Here's how the part is built. I have some questions about the finished solid (model axes, mm). A direction names the side the tool comes from. Give positions to 0.01 mm unless a question says otherwise; leave off trailing zeros. Loops run counter-clockwise (first coordinate to the right, second up) from the corner with the lowest first, then second, coordinate; pieces in that order, holes last.
Q1. If we section it at A-A (z = 0): Please give me the cut outline in (x, y), plus the area to 3 significant figures.
Q2. I need wall thicknesses on line 1 (Z direction, x = 6, y = -13); line 2 (X direction, y = -6.75, z = 9.5); line 3 (Y direction, x = 23.5, z = 13). Which ranges of each line are inside material? Lowest first, please.
Q3. If we section it at B-B (y = -14.5): Please give me the cut outline in (x, z).
Q4. Will these pins go through, and if not, where does the flat tip stop? P1, Ø4, axis at x = 6, z = 34, coming from the -Y side; P2, Ø0.9, axis at x = 23.5, y = 1.5, coming from the +Z side.
Q5. For faces 1 (the face through (-26, -10.8, -43.57)), 2 (the face through (0, -12, -42.5)), 3 (the face through (25.273, 1, 0)), 4 (the face through (20.273, 1, 0)), which set-ups out of +Z, -Z, +X, -X, +Y, -Y let a thin tool reach every point of the face, with its end or its side?
Q6. If we section it at D-D (y = 1.25): Please give me the cut outline in (x, z), plus the area to 3 significant figures.
Q7. If we section it at C-C (x = 13): Please give me the cut outline in (y, z).
Q8. We'd pull the mould along X, two halves only. Please class faces 5 (the face through (18.677, 1.479, -17.722)), 6 (the face through (-27, -25, 0)), 7 (the face through (-27.5, -11, 1)): +X half, -X half, draft (parallel to the pull), parting line (faces both ways), or undercut.
Autodesk Inventor part; units mm, degrees
ref_plane "YZ Plane" through (0, 0, 0) normal (1, 0, 0) x (0, 1, 0)
ref_plane "XZ Plane" through (0, 0, 0) normal (0, 1, 0) x (-1, 0, 0)
ref_plane "XY Plane" through (0, 0, 0) normal (0, 0, 1) x (1, 0, 0)
sketch "Sketch1" plane through (0, 0, 0) normal (0, 1, 0) x (-1, 0, 0)
  line L0 (22.5, 45) -> (-22.5, 45)
  line L1 (-27.5, 40) -> (-27.5, -40)
  line L2 (-22.5, -45) -> (22.5, -45)
  line L3 (27.5, -40) -> (27.5, 40)
  line L4 (27.5, 45) -> (-27.5, -45) construction
  line L5 (-27.5, 45) -> (27.5, -45) construction
  line L6 (0, 0) -> (17.6777, 17.6777) construction
  line L7 (0, 0) -> (25, 0) construction
  circle A0 centre (17.6777, 17.6777) radius 1
  line L8 (17.6777, 17.6777) -> (21.2132, 14.1421) construction
  arc A1 (21.2132, 14.1421) -> (14.1421, 21.2132) centre (17.6777, 17.6777) ccw construction
  circle A2 centre (0, 0) radius 20 construction
  line L9 (14.1421, 21.2132) -> (10.1575, 17.2286) construction
  arc A3 (-6.25, 18.9984) -> (6.25, 18.9984) centre (0, 0) ccw construction
  line L10 (21.2132, 14.1421) -> (17.2286, 10.1575) construction
  line L11 (-14.1421, 21.2132) -> (-10.1575, 17.2286) construction
  arc A4 (-14.1421, 21.2132) -> (-21.2132, 14.1421) centre (-17.6777, 17.6777) ccw construction
  line L12 (-21.2132, 14.1421) -> (-17.2286, 10.1575) construction
  circle A5 centre (-17.6777, 17.6777) radius 1
  line L13 (-21.2132, -14.1421) -> (-17.2286, -10.1575) construction
  arc A6 (-21.2132, -14.1421) -> (-14.1421, -21.2132) centre (-17.6777, -17.6777) ccw construction
  line L14 (-14.1421, -21.2132) -> (-10.1575, -17.2286) construction
  circle A7 centre (-17.6777, -17.6777) radius 1
  line L15 (14.1421, -21.2132) -> (10.1575, -17.2286) construction
  arc A8 (14.1421, -21.2132) -> (21.2132, -14.1421) centre (17.6777, -17.6777) ccw construction
  line L16 (21.2132, -14.1421) -> (17.2286, -10.1575) construction
  circle A9 centre (17.6777, -17.6777) radius 1
  line L17 (-20.273, 10) -> (-25.273, 10)
  line L18 (-25.273, 10) -> (-25.273, -10)
  line L19 (-25.273, -10) -> (-20.273, -10)
  line L20 (-20.273, -10) -> (-20.273, 10)
  line L21 (-20.273, 10) -> (-25.273, -10) construction
  line L22 (-25.273, 10) -> (-20.273, -10) construction
  line L23 (39.9497, 0) -> (-39.9497, 0)
  arc A10 (22.5, -45) -> (27.5, -40) centre (22.5, -40) ccw
  arc A11 (27.5, 40) -> (22.5, 45) centre (22.5, 40) ccw
  arc A12 (-22.5, 45) -> (-27.5, 40) centre (-22.5, 40) ccw
  arc A13 (-27.5, -40) -> (-22.5, -45) centre (-22.5, -40) ccw
  point P0 (-22.773, 0)
  point P1 (-22.773, 0)
  dimension "d0" = 55
  dimension "d1" = 90
  dimension "d4" = 25
  dimension "d5" = 45
  dimension "d6" = 2
  dimension "d7" = 5
  dimension "d8" = 360
  dimension "d9" = 5
  dimension "d10" = 20
  dimension "d18" = 5
extrude "Extrusion1" add sketch "Sketch1" along normal blind 3 contours A11 L3 L23 L20 L17 L18 L1 A12 L0 | L3 A10 L2 A13 L1 L23 L18 L19 L20
sketch "Sketch2" plane through (0, 0, 0) normal (0, -1, 0) x (1, 0, 0)
  line L0 (22.5, 45) -> (-22.5, 45)
  line L1 (-27.5, 40) -> (-27.5, -40)
  line L2 (-22.5, -45) -> (22.5, -45)
  line L3 (27.5, -40) -> (27.5, 40)
  line L4 (27.5, 45) -> (-27.5, -45) construction
  line L5 (-27.5, 45) -> (27.5, -45) construction
  line L6 (17, 42.5) -> (-17, 42.5)
  line L7 (-25, 34.5) -> (-25, -34.5)
  line L8 (-17, -42.5) -> (17, -42.5)
  line L9 (25, -34.5) -> (25, 34.5)
  line L10 (25, 42.5) -> (-25, -42.5) construction
  line L11 (-25, 42.5) -> (25, -42.5) construction
  arc A0 (25, 34.5) -> (17, 42.5) centre (17, 34.5) ccw
  arc A1 (17, -42.5) -> (25, -34.5) centre (17, -34.5) ccw
  arc A2 (-25, -34.5) -> (-17, -42.5) centre (-17, -34.5) ccw
  arc A3 (-17, 42.5) -> (-25, 34.5) centre (-17, 34.5) ccw
  arc A4 (27.5, 40) -> (22.5, 45) centre (22.5, 40) ccw
  arc A5 (-22.5, 45) -> (-27.5, 40) centre (-22.5, 40) ccw
  arc A6 (-27.5, -40) -> (-22.5, -45) centre (-22.5, -40) ccw
  arc A7 (22.5, -45) -> (27.5, -40) centre (22.5, -40) ccw
  point P0 (0, 0)
  dimension "d13" = 55
  dimension "d14" = 90
  dimension "d15" = 50
  dimension "d16" = 85
  dimension "d17" = 8
  dimension "d21" = 5
extrude "Extrusion2" add sketch "Sketch2" along normal blind 25
properties part number "mount1"
Check sheet entries:
1. outline: (-27.5, -25) - (-25, -25) - (-25, 0) - (20.27, 0) - (20.27, 3) - (-27.5, 3) - close; (25, -25) - (27.5, -25) - (27.5, 3) - (25.27, 3) - (25.27, 0) - (25, 0) - close
1. area: 275 mm2
2. line 1: z = -45 to -42.5, 42.5 to 45
2. line 2: x = -27.5 to -25, 25 to 27.5
2. line 3: y = 0 to 3
3. outline: (-27.5, -40) arc R5 ccw to (-22.5, -45) - (22.5, -45) arc R5 ccw to (27.5, -40) - (27.5, 40) arc R5 ccw to (22.5, 45) - (-22.5, 45) arc R5 ccw to (-27.5, 40) - close; hole (-25, -34.5) arc R8 ccw to (-17, -42.5) - (17, -42.5) arc R8 ccw to (25, -34.5) - (25, 34.5) arc R8 ccw to (17, 42.5) - (-17, 42.5) arc R8 ccw to (-25, 34.5) - close
4. P1: stops at y = 0
4. P2: stops at z = 44.97
5. face 1: -Z, -X, +Y, -Y
5. face 2: -Y
5. face 3: +Y
5. face 4: +Y, -Y
6. outline: (-27.5, -40) arc R5 ccw to (-22.5, -45) - (22.5, -45) arc R5 ccw to (27.5, -40) - (27.5, 40) arc R5 ccw to (22.5, 45) - (-22.5, 45) arc R5 ccw to (-27.5, 40) - close; hole circle Ø2 at (-17.68, -17.68); hole circle Ø2 at (-17.68, 17.68); hole circle Ø2 at (17.68, -17.68); hole circle Ø2 at (17.68, 17.68); hole (20.27, -10) - (25.27, -10) - (25.27, 10) - (20.27, 10) - close
6. area: 4,820 mm2
7. outline: (-25, -45) - (3, -45) - (3, 45) - (-25, 45) - (-25, 42.5) - (0, 42.5) - (0, -42.5) - (-25, -42.5) - close
8. face 5: undercut
8. face 6: draft
8. face 7: -X half
